Autodesk Fusion 360 part; units mm, degrees
sketch "Sketch1" plane through (0, 0, 0) normal (0, 0, 1) x (1, 0, 0)
  line L0 (4, 4.645) -> (4, 6.9613)
  line L1 (8, 10.9613) -> (12, 10.9613)
  line L2 (16, 6.9613) -> (16, 2.9855)
  line L3 (13, 2) -> (15, 2)
  line L4 (15, 2.9855) -> (15, 6.9613)
  line L5 (12, 9.9613) -> (7.8172, 9.9613)
  line L6 (17, 1.9855) -> (19, 1.9855)
  arc A0 (16, 2.9855) -> (17, 1.9855) centre (17, 2.9855) ccw
  line L7 (14, 1.9855) -> (1, 1.9855)
  arc A1 (14, 1.9855) -> (15, 2.9855) centre (14, 2.9855) ccw
  line L8 (0, 0.9855) -> (0, 0)
  line L9 (0, 0) -> (20, 0)
  line L10 (20, 0) -> (20, 0.9855)
  arc A2 (1, 1.9855) -> (0, 0.9855) centre (1, 0.9855) ccw
  arc A3 (20, 0.9855) -> (19, 1.9855) centre (19, 0.9855) ccw
  arc A4 (4, 4.645) -> (4.8517, 5.6339) centre (5, 4.645) ccw
  arc A5 (8, 10.9613) -> (4, 6.9613) centre (8, 6.9613) ccw
  arc A6 (16, 6.9613) -> (12, 10.9613) centre (12, 6.9613) ccw
  arc A7 (7.8172, 9.9613) -> (4.8173, 6.9821) centre (7.8172, 6.9613) ccw
  arc A8 (15, 6.9613) -> (12, 9.9613) centre (12, 6.9613) ccw
  line L11 (4.8173, 6.9821) -> (4.8517, 5.6339)
  dimension "d5" = 1
  dimension "d6" = 1
  dimension "d9" = 1
  dimension "d10" = 1
  dimension "d12" = 1
  dimension "d13" = 1
  dimension "d14" = 4
  dimension "d15" = 4
  dimension "d16" = 20
  dimension "d21" = 1
  dimension "d23" = 4
  dimension "d24" = 4
  dimension "d25" = 3
  dimension "d26" = 3
extrude "Extrude1" add sketch "Sketch1" along normal blind 10
Verification items for the finished model (mm, model axes). A direction names the side the tool comes from. Give positions to 0.01 mm unless a question says otherwise; leave off trailing zeros. Order: outer loops, then holes, each group sorted by start corner. A loop starts at its lowest first (then second) coordinate and runs counter-clockwise, first axis right, second up. Notation, with made-up numbers: (-19, -11.75) -> (6, -11.75) arc R24 ccw to (6, 7.25) -> close; hole circle Ø6 at (-1, 6). An arc over 180 degrees is marked (long way). One line per item, written item: value.
(1) Sectioned sample at C-C on z = 8.25. Record the cut outline in (x, y) (1 decimal), then the cut area to 3 significant figures.
Final values:
outline: (0, 0) -> (20, 0) -> (20, 1) arc R1 ccw to (19, 2) -> (17, 2) arc R1 cw to (16, 3) -> (16, 7) arc R4 ccw to (12, 11) -> (8, 11) arc R4 ccw to (4, 7) -> (4, 4.6) arc R1 ccw (long way) to (4.9, 5.6) -> (4.8, 7) arc R3 cw to (7.8, 10) -> (12, 10) arc R3 cw to (15, 7) -> (15, 3) arc R1 cw to (14, 2) -> (1, 2) arc R1 ccw to (0, 1) -> close
area: 63.6 mm^2
(2) Scan lines: line 1 along X through (y, z) = (6.75, 9); line 2 along Y through (x, z) = (10, 0.5); line 3 along X through (y, z) = (3, 6.75). Record each from-to range of solid material in increasing order. Write a range as [from, to].
Final values:
line 1: [4, 4.82], [15, 16]
line 2: [0, 1.99], [9.96, 10.96]
line 3: [15, 16]
(3) Draft check along Y on faces 1 (the face through (10, 1, 10)), 2 (the face through (15, 5, 5)), 3 (the face through (10, 0, 5)). Enter one of: pulls with the +Y half, pulls with the -Y half, needs draft (parallel to the pull), parting line crosses it, or undercut.
Final values:
face 1: needs draft
face 2: undercut
face 3: pulls with the -Y half
(4) Gauge pin test, flat ends, axial feed: pin 1 (2.5 mm diameter, centred on y = 6.5, z = 5, fed in from -X); pin 2 (4 mm diameter, centred on y = 5, z = 3.5, fed in from +X); pin 3 (1 mm diameter, centred on x = 7, z = 7, fed in from +Y). Record the tip position at first contact, or that the pin passes through.
Final values:
pin 1: x = 4
pin 2: x = 16
pin 3: y = 10.93
(5) Sectioned sample at A-A on x = 8.5. Record the cut outline in (y, z).
Final values:
outline: (0, 0) -> (1.99, 0) -> (1.99, 10) -> (0, 10) -> close; (9.96, 0) -> (10.96, 0) -> (10.96, 10) -> (9.96, 10) -> close
(6) Sectioned sample at B-B on x = 5.25. Record the cut outline in (y, z).
Final values:
outline: (0, 0) -> (1.99, 0) -> (1.99, 10) -> (0, 10) -> close; (3.68, 0) -> (5.61, 0) -> (5.61, 10) -> (3.68, 10) -> close; (8.51, 0) -> (9.87, 0) -> (9.87, 10) -> (8.51, 10) -> close
(7) Sectioned sample at D-D on x = 12.25. Record the cut outline in (y, z), then the cut area to 3 significant figures.
Final values:
outline: (0, 0) -> (1.99, 0) -> (1.99, 10) -> (0, 10) -> close; (9.95, 0) -> (10.95, 0) -> (10.95, 10) -> (9.95, 10) -> close
area: 29.9 mm^2
(8) Tool access check on faces 4 (the face through (8, 1.986, 5)), 5 (the face through (5.68, 9.067, 4.93)), 6 (the face through (18, 1.986, 5)), 7 (the face through (4, 6, 5)). Record the directions out of +Z, -Z, +X, -X, +Y, -Y that give a thin tool (end or side, any length) a straight path to the whole face; none if there is none.
Final values:
face 4: +Z, -Z, -X
face 5: +Z, -Z
face 6: +Z, -Z, +X, +Y
face 7: +Z, -Z, -X, +Y
